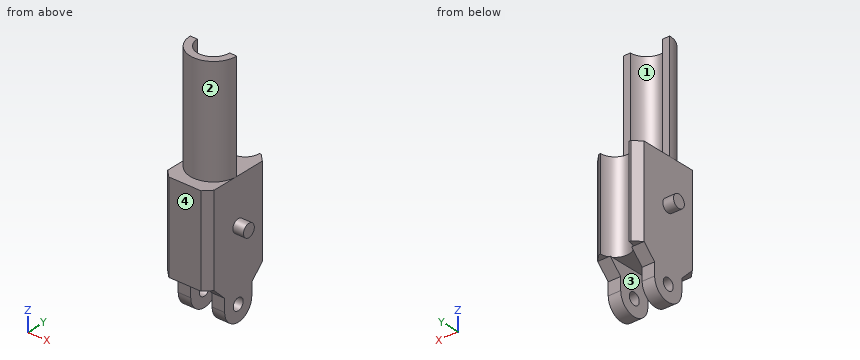
```python
from build123d import *

# Parameters (mm, degrees)
BOSS_EXTRUDE1_DEPTH     = 30
SKETCH2_W               = 13
SKETCH2_H               = 20
BOSS_EXTRUDE2_DEPTH     = 25
CHAMFER1_SIZE           = 2
SKETCH3_R               = 4
CUT_EXTRUDE1_DEPTH      = 40
SKETCH4_R               = 1.8
BOSS_EXTRUDE3_DEPTH     = 9.5
BOSS_EXTRUDE4_REACH     = 37.584
SKETCH5_R               = 1.65
CUT_EXTRUDE2_DEPTH      = 41.40730132
CUT_EXTRUDE2_DEPTH_BACK = 41.40730132
SKETCH6_W               = 6
SKETCH6_H               = 11.5


with BuildPart() as part:
    # Sketch1 → Boss-Extrude1 (new body)
    with BuildSketch(Plane.XY):
        with BuildLine():
            Line((6.5, 0), (4.5, 0))
            ThreePointArc((4.5, 0), (0, -4.5), (-4.5, 0))
            Line((-4.5, 0), (-6.5, 0))
            ThreePointArc((-6.5, 0), (0, -6.5), (6.5, 0))
        make_face()
    extrude(amount=BOSS_EXTRUDE1_DEPTH)

    # Sketch2 → Boss-Extrude2 (add)
    with BuildSketch(Plane(origin=(0, 0, 0), x_dir=(-1, 0, 0), z_dir=(0, 0, -1))):
        with Locations((0, 0.5)):
            Rectangle(SKETCH2_W, SKETCH2_H)
    extrude(amount=BOSS_EXTRUDE2_DEPTH)

    # Chamfer1
    chamfer1_edges = [part.edges().sort_by_distance(p)[0] for p in [
        (6.5, 10.5, -12.5),
        (6.5, -9.5, -12.5),
        (-6.5, -9.5, -12.5),
        (-6.5, 10.5, -12.5),
    ]]
    chamfer(chamfer1_edges, length=CHAMFER1_SIZE)

    # Sketch3 → Cut-Extrude1 (cut)
    with BuildSketch(Plane(origin=(0, 0, -25), x_dir=(-1, 0, 0), z_dir=(0, 0, -1))):
        with Locations((0, 10.5)):
            Circle(SKETCH3_R)
    extrude(amount=-CUT_EXTRUDE1_DEPTH, mode=Mode.SUBTRACT)

    # Sketch4 → Boss-Extrude3 (add, symmetric)
    with BuildSketch(Plane(origin=(0, 0, 0), x_dir=(0, 0, -1), z_dir=(1, 0, 0))):
        with Locations(Location((12.5, 0.5, 0), (0, 0, 90))):
            Circle(SKETCH4_R)
    extrude(amount=BOSS_EXTRUDE3_DEPTH, both=True)

    # Boss-Extrude4: up to this face of the body (flat: up to its plane)
    boss_extrude4_end = Plane(part.part.faces().sort_by_distance((-6.5, -3.75, -0.296816442))[0])
    # Sketch5 → Boss-Extrude4 (add, up to the picked face)
    with BuildSketch(Plane(origin=(6.5, 0, 0), x_dir=(0, 0, -1), z_dir=(1, 0, 0)), mode=Mode.PRIVATE) as boss_extrude4_sk1:
        with BuildLine():
            Line((32, 5), (28.5, 5))
            Line((28.5, 5), (25, 8.5))
            Line((25, 8.5), (25, -7.5))
            Line((25, -7.5), (28.5, -4))
            Line((28.5, -4), (32, -4))
            ThreePointArc((32, -4), (36.5, 0.5), (32, 5))
        make_face()
        with Locations(Location((32, 0.5, 0), (0, 0, 90))):
            Circle(SKETCH5_R, mode=Mode.SUBTRACT)
    boss_extrude4_tool1 = split(extrude(boss_extrude4_sk1.sketch, amount=-BOSS_EXTRUDE4_REACH, mode=Mode.PRIVATE), bisect_by=boss_extrude4_end, keep=Keep.BOTH, mode=Mode.PRIVATE)
    add(boss_extrude4_tool1.solids().sort_by(Axis((6.5, 0.5, -29.652842), (-1, 0, 0)))[0])

    # Sketch6 → Cut-Extrude2 (cut, two sides: drawn at the far end of the back side and taken through both)
    with BuildSketch(Plane(origin=(0, 5, 0), x_dir=(1, 0, 0), z_dir=(0, 1, 0)).offset(-CUT_EXTRUDE2_DEPTH_BACK)):
        with Locations((0, 30.75)):
            Rectangle(SKETCH6_W, SKETCH6_H)
    extrude(amount=CUT_EXTRUDE2_DEPTH + CUT_EXTRUDE2_DEPTH_BACK, mode=Mode.SUBTRACT)


solid = part.part
```
Verification items for the finished model (mm, model axes). Face numbers are marked on the shaded views. A direction names the side the tool comes from. Round coordinates to 2 decimals unless told otherwise and drop trailing zeros. Loops run counter-clockwise (first coordinate to the right, second up) from the corner with the lowest first, then second, coordinate; pieces in that order, holes last. Notation, with made-up numbers: (14.25, -26) -> (37.25, -26) arc R17 ccw to (37.25, -11) -> close; hole circle Ø6 at (44, 31). An arc over 180 degrees is marked (long way). Answer as a JSON object with one key per item and string values.
Q1. Go/stop test with flat-tipped pins: P1, Ø4, axis at y = 0.5, z = -32, coming from the -X side; P2, Ø3, axis at x = -4.5, z = 14, coming from the +Y side; P3, Ø10, axis at x = 2, z = -15.5, coming from the +Y side; P4, Ø4, axis at x = 1, z = 20.5, coming from the +Y side. Record where each tip stops, or that it passes through.
Data:
{"P1": "stops at x = -6.5", "P2": "stops at y = 0", "P3": "stops at y = 10.5", "P4": "stops at y = -3.35"}
Q2. Section check B-B (z = -12.5). Record the boundary of the cut face in (x, y).
Data:
{"outline": "(-9.5, -1.3) -> (-6.5, -1.3) -> (-6.5, -7.5) -> (-4.5, -9.5) -> (4.5, -9.5) -> (6.5, -7.5) -> (6.5, -1.3) -> (9.5, -1.3) -> (9.5, 2.3) -> (6.5, 2.3) -> (6.5, 8.5) -> (4.5, 10.5) -> (4, 10.5) arc R4 cw to (-4, 10.5) -> (-4.5, 10.5) -> (-6.5, 8.5) -> (-6.5, 2.3) -> (-9.5, 2.3) -> close"}
Q3. Section check A-A (z = -26). Record the boundary of the cut face in (x, y).
Data:
{"outline": "(-6.5, -6.5) -> (-3, -6.5) -> (-3, 7.5) -> (-6.5, 7.5) -> close; (3, -6.5) -> (6.5, -6.5) -> (6.5, 7.5) -> (3, 7.5) -> close"}
Q4. Access from +Z, -Z, +X, -X, +Y, -Y to the whole of each face (thin tool, end or side, straight path). Record for the marked faces 1, 2, 3 and 4.
Data:
{"face 1": "+Z, +Y", "face 2": "+Z, -Y", "face 3": "-Z, +Y, -Y", "face 4": "+Z, -Z, +X, -X, -Y"}
Q5. Section check C-C (x = 1.5). Record the boundary of the cut face in (y, z).
Data:
{"outline": "(-9.5, -25) -> (6.79, -25) -> (6.79, 0) -> (-4.24, 0) -> (-4.24, 30) -> (-6.32, 30) -> (-6.32, 0) -> (-9.5, 0) -> close"}
Q6. Scan lines: line 1 (Z direction, x = -4.75, y = 0.5); line 2 (Y direction, x = 0.25, z = 11); line 3 (X direction, y = 3.75, z = -2). Record each from-to range of solid material in increasing order. Write a range as from..to.
Data:
{"line 1": "z = -36.5..-33.65, -30.35..0", "line 2": "y = -6.5..-4.49", "line 3": "x = -6.5..6.5"}
Q7. Section check D-D (y = -8.5). Record the boundary of the cut face in (x, z).
Data:
{"outline": "(-5.5, -25) -> (5.5, -25) -> (5.5, 0) -> (-5.5, 0) -> close"}
